```python
from build123d import *

# Parameters (mm, degrees)
SKETCH8_W           = 203.2
SKETCH8_H           = 63.5
BOSS_EXTRUDE1_DEPTH = 6.35
SKETCH9_R           = 14.2875
CUT_EXTRUDE2_DEPTH  = 1.5875
SKETCH10_R          = 6.35
CUT_EXTRUDE3_DEPTH  = 5.7625
SKETCH11_R          = 6.35
CUT_EXTRUDE4_DEPTH  = 7.35


with BuildPart() as part:
    # Sketch8 → Boss-Extrude1 (new body)
    with BuildSketch(Plane(origin=(0, 0, 0), x_dir=(1, 0, 0), z_dir=(0, 1, 0))):
        with Locations((-101.6, 31.75)):
            Rectangle(SKETCH8_W, SKETCH8_H)
    extrude(amount=BOSS_EXTRUDE1_DEPTH)

    # Sketch9 → Cut-Extrude2 (cut)
    with BuildSketch(Plane(origin=(0, 6.35, 0), x_dir=(1, 0, 0), z_dir=(0, 1, 0))):
        with Locations((-101.6, 31.75)):
            Circle(SKETCH9_R)
    extrude(amount=-CUT_EXTRUDE2_DEPTH, mode=Mode.SUBTRACT)

    # Sketch10 → Cut-Extrude3 (cut, through all)
    with BuildSketch(Plane(origin=(0, 4.7625, 0), x_dir=(1, 0, 0), z_dir=(0, 1, 0))):
        with Locations((-101.6, 31.75)):
            Circle(SKETCH10_R)
    extrude(amount=-CUT_EXTRUDE3_DEPTH, mode=Mode.SUBTRACT)

    # Sketch11 → Cut-Extrude4 (cut, through all)
    with BuildSketch(Plane(origin=(0, 6.35, 0), x_dir=(1, 0, 0), z_dir=(0, 1, 0))):
        with Locations((-171.45, 31.75)):
            Circle(SKETCH11_R)
        with Locations((-31.75, 31.75)):
            Circle(SKETCH11_R)
    extrude(amount=-CUT_EXTRUDE4_DEPTH, mode=Mode.SUBTRACT)


solid = part.part
```
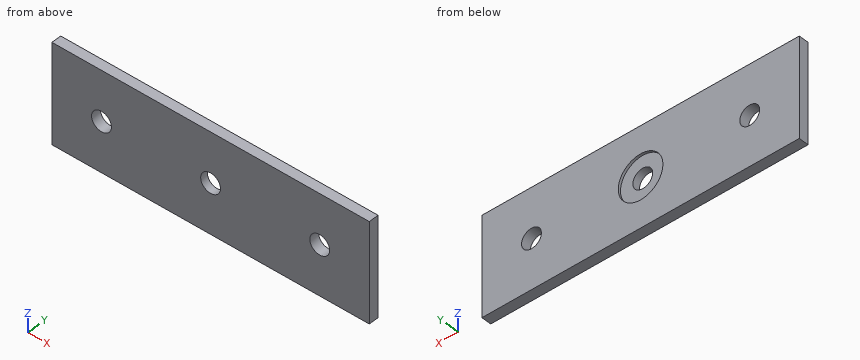
The model under review builds one solid part; all positions refer to its coordinate system, in mm. Coordinates: 2 decimals unless noted, no trailing zeros. Write each loop counter-clockwise with the first axis right and the second up, starting at its lowest first coordinate (ties: lowest second). Pieces come first, ordered by that corner, then holes.
1) We need section A-A on x = -31.75. State the section outline as (y, z) points.
2) We need section C-C on y = 3.25. State the section outline as (x, z) points, then the cut area to 3 significant figures.
3) To check wall thickness, follow probe 1 along X at (y, z) = (1.95, -31.75); probe 2 along Z at (x, y) = (-171.45, 1.75); probe 3 along X at (y, z) = (5, -31.75). State the ranges of each line that lie inside material, in increasing order.
4) We need section B-B on z = -31.75. State the section outline as (x, y) points, then the cut area to 3 significant figures.
5) We need section D-D on x = -101.6. State the section outline as (y, z) points, then the cut area to 3 significant figures.
6) Clearance check with a flat-ended pin moving along its axis: pin 1 Ø23 at (x, z) = (-101.6, -31.75) entering from +Y. State where the tip first meets the part, or that it passes through.
Answer list:
1. outline: (0, -63.5) - (6.35, -63.5) - (6.35, -38.1) - (0, -38.1) - close; (0, -25.4) - (6.35, -25.4) - (6.35, 0) - (0, 0) - close
2. outline: (-203.2, -63.5) - (0, -63.5) - (0, 0) - (-203.2, 0) - close; hole circle Ø12.7 at (-171.45, -31.75); hole circle Ø12.7 at (-101.6, -31.75); hole circle Ø12.7 at (-31.75, -31.75)
2. area: 12,500 mm2
3. probe 1: x = -203.2 to -177.8, -165.1 to -107.95, -95.25 to -38.1, -25.4 to 0
3. probe 2: z = -63.5 to -38.1, -25.4 to 0
3. probe 3: x = -203.2 to -177.8, -165.1 to -115.89, -87.31 to -38.1, -25.4 to 0
4. outline: (-203.2, 0) - (-177.8, 0) - (-177.8, 6.35) - (-203.2, 6.35) - close; (-165.1, 0) - (-107.95, 0) - (-107.95, 4.76) - (-115.89, 4.76) - (-115.89, 6.35) - (-165.1, 6.35) - close; (-95.25, 0) - (-38.1, 0) - (-38.1, 6.35) - (-87.31, 6.35) - (-87.31, 4.76) - (-95.25, 4.76) - close; (-25.4, 0) - (0, 0) - (0, 6.35) - (-25.4, 6.35) - close
4. area: 1,020 mm2
5. outline: (0, -63.5) - (6.35, -63.5) - (6.35, -46.04) - (4.76, -46.04) - (4.76, -38.1) - (0, -38.1) - close; (0, -25.4) - (4.76, -25.4) - (4.76, -17.46) - (6.35, -17.46) - (6.35, 0) - (0, 0) - close
5. area: 297 mm2
6. pin 1: stops at y = 4.76
